```python
from build123d import *

# Parameters (mm, degrees)
F0_W     = 13
F0_H     = 4
F0_W_2   = 12
F1_DEPTH = 5
F2_DEPTH = 9
F4_DEPTH = 4


with BuildPart() as f1:
    # F0 (on Top) → F1 (new body)
    with BuildSketch(Plane.XY):
        with Locations((6.5, 2)):
            Rectangle(F0_W, F0_H)
        with Locations((19, 2)):
            Rectangle(F0_W_2, F0_H)
        with Locations((31.5, 2)):
            Rectangle(F0_W, F0_H)
        with Locations((44, 2)):
            Rectangle(F0_W_2, F0_H)
        with Locations((56.5, 2)):
            Rectangle(F0_W, F0_H)
        with Locations((69, 2)):
            Rectangle(F0_W_2, F0_H)
        with Locations((81.5, 2)):
            Rectangle(F0_W, F0_H)
        with Locations((94, 2)):
            Rectangle(F0_W_2, F0_H)
        with Locations((106.5, 2)):
            Rectangle(F0_W, F0_H)
        with Locations((119, 2)):
            Rectangle(F0_W_2, F0_H)
        with Locations((131.5, 2)):
            Rectangle(F0_W, F0_H)
    extrude(amount=F1_DEPTH)

    # F0 (on Top) → F2 (join)
    with BuildSketch(Plane.XY):
        with Locations((6.5, 2)):
            Rectangle(F0_W, F0_H)
        with Locations((31.5, 2)):
            Rectangle(F0_W, F0_H)
        with Locations((56.5, 2)):
            Rectangle(F0_W, F0_H)
        with Locations((81.5, 2)):
            Rectangle(F0_W, F0_H)
        with Locations((106.5, 2)):
            Rectangle(F0_W, F0_H)
        with Locations((131.5, 2)):
            Rectangle(F0_W, F0_H)
    extrude(amount=F2_DEPTH)

    # F3 (on face) → F4 (join)
    with BuildSketch(Plane.XZ):
        Polygon((13, 0), (0, 0), (6.5, -18.91428), align=None)
        Polygon((38, 0), (25, 0), (31.5, -18.91428), align=None)
        Polygon((63, 0), (50, 0), (56.5, -18.91428), align=None)
        Polygon((88, 0), (75, 0), (81.5, -18.91428), align=None)
        Polygon((113, 0), (100, 0), (106.5, -18.91428), align=None)
        Polygon((138, 0), (125, 0), (131.5, -18.91428), align=None)
    extrude(amount=-F4_DEPTH)


solid = f1.part
```
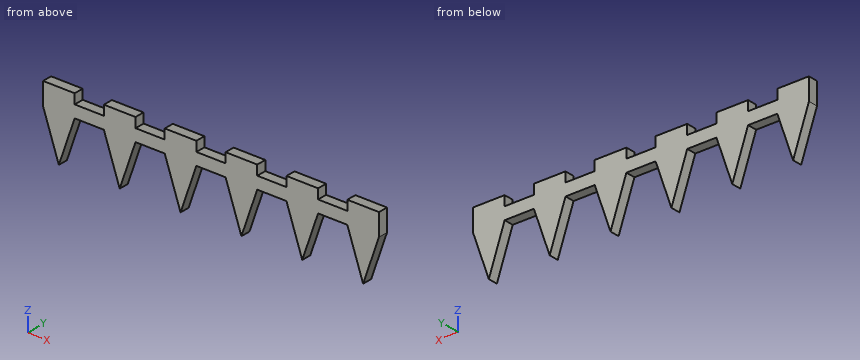
Geometry check sheet. Reference: the model listing, model coordinates, mm. Round coordinates to 2 decimals unless told otherwise and drop trailing zeros. Order: outer loops, then holes, each group sorted by start corner. A loop starts at its lowest first (then second) coordinate and runs counter-clockwise, first axis right, second up. Notation, with made-up numbers: (4.5, 10) -> (29.5, 10) arc R33 ccw to (29.5, 39) -> close; hole circle Ø1 at (26, -40). An arc over 180 degrees is marked (long way). Return JSON: item names as keys, results as strings. Group by question number.
Q1. Section check A-A, the plane z = 6.5. Record the boundary of the cut face in (x, y), plus the area to 3 significant figures.
Q2. Section check B-B, the plane x = 43.5. Record the boundary of the cut face in (y, z), plus the area to 3 significant figures.
Q3. Section check C-C, the plane z = -6. Record the boundary of the cut face in (x, y), plus the area to 3 significant figures.
Q4. Material ranges on probe 1 along X at (y, z) = (1.55, 5.75); probe 2 along X at (y, z) = (3.65, -14.75); probe 3 along Z at (x, y) = (89.5, 0.35), recorded low to high. Write a range as from..to.
Q5. Section check D-D, the plane x = 110.5. Record the boundary of the cut face in (y, z), plus the area to 3 significant figures.
Q6. Gauge pin test, flat ends, axial feed: pin 1 (2 mm diameter, centred on x = 119.5, y = 3, fed in from -Z); pin 2 (2 mm diameter, centred on x = 16.5, y = 2, fed in from +Z). Record the tip position at first contact, or that the pin passes through.
Numbers:
{
 "1": {"outline": "(0, 0) -> (13, 0) -> (13, 4) -> (0, 4) -> close; (25, 0) -> (38, 0) -> (38, 4) -> (25, 4) -> close; (50, 0) -> (63, 0) -> (63, 4) -> (50, 4) -> close; (75, 0) -> (88, 0) -> (88, 4) -> (75, 4) -> close; (100, 0) -> (113, 0) -> (113, 4) -> (100, 4) -> close; (125, 0) -> (138, 0) -> (138, 4) -> (125, 4) -> close", "area": "312 mm^2"},
 "2": {"outline": "(0, 0) -> (4, 0) -> (4, 5) -> (0, 5) -> close", "area": "20.0 mm^2"},
 "3": {"outline": "(2.06, 0) -> (10.94, 0) -> (10.94, 4) -> (2.06, 4) -> close; (27.06, 0) -> (35.94, 0) -> (35.94, 4) -> (27.06, 4) -> close; (52.06, 0) -> (60.94, 0) -> (60.94, 4) -> (52.06, 4) -> close; (77.06, 0) -> (85.94, 0) -> (85.94, 4) -> (77.06, 4) -> close; (102.06, 0) -> (110.94, 0) -> (110.94, 4) -> (102.06, 4) -> close; (127.06, 0) -> (135.94, 0) -> (135.94, 4) -> (127.06, 4) -> close", "area": "213 mm^2"},
 "4": {"probe 1": "0..13, 25..38, 50..63, 75..88, 100..113, 125..138", "probe 2": "5.07..7.93, 30.07..32.93, 55.07..57.93, 80.07..82.93, 105.07..107.93, 130.07..132.93", "probe 3": "0..5"},
 "5": {"outline": "(0, -7.27) -> (4, -7.27) -> (4, 9) -> (0, 9) -> close", "area": "65.1 mm^2"},
 "6": {"pin 1": "z = 0", "pin 2": "z = 5"}
}
